Could you check a few things on this model? Use its own coordinates, in mm. A direction names the side the tool comes from. Round coordinates to 2 decimals unless told otherwise and drop trailing zeros. Use CSV: the item, a comma, the result in double quotes. Start each with the question number.
Autodesk Inventor part; units mm, degrees
ref_plane "Work Plane1" through (-41.275, 69.85, 0) normal (0, -1, 0) x (0, 0, -1)
ref_plane "YZ Plane" through (0, 0, 0) normal (1, 0, 0) x (0, 1, 0)
ref_plane "XZ Plane" through (0, 0, 0) normal (0, 1, 0) x (-1, 0, 0)
sketch "Sketch1" plane through (0, 0, 0) normal (0, 0, 1) x (1, 0, 0)
  line L0 (-47.625, -69.85) -> (47.625, -69.85)
  line L1 (47.625, -69.85) -> (47.625, 69.85)
  line L2 (47.625, 69.85) -> (-47.625, 69.85)
  line L3 (-47.625, 69.85) -> (-47.625, -69.85)
  line L4 (-47.625, -69.85) -> (47.625, 69.85) construction
  line L5 (47.625, -69.85) -> (-47.625, 69.85) construction
  point P0 (0, 0)
  dimension "d2" = 95.25
  dimension "d3" = 139.7
extrude "Extrusion1" add sketch "Sketch1" along normal blind 12.7
sketch "Sketch5" plane through (0, 0, 0) normal (0, 0, -1) x (-1, 0, 0)
  circle A0 centre (68.072, -112.9665) radius 2.5527
  circle A1 centre (17.272, -112.9665) radius 2.5527
  circle A2 centre (-33.528, -112.9665) radius 2.5527
  circle A3 centre (-84.328, -112.9665) radius 2.5527
  circle A4 centre (-135.128, -112.9665) radius 2.5527
  circle A5 centre (-185.928, -112.9665) radius 2.5527
  circle A6 centre (-211.328, -112.9665) radius 2.5527
  circle A7 centre (-160.528, -112.9665) radius 2.5527
  circle A8 centre (-109.728, -112.9665) radius 2.5527
  circle A9 centre (-58.928, -112.9665) radius 2.5527
  circle A10 centre (-8.128, -112.9665) radius 2.5527
  circle A11 centre (42.672, -112.9665) radius 2.5527
  circle A12 centre (93.472, -112.9665) radius 2.5527
  circle A13 centre (-62.484, -38.6715) radius 3.429
  circle A14 centre (-62.484, 33.7185) radius 3.429
  arc A15 (-54.102, -15.1765) -> (-44.45, -15.1765) centre (-49.276, -15.1765) ccw
  line L0 (-44.45, -15.1765) -> (-44.45, 10.2235)
  arc A16 (-44.45, 10.2235) -> (-54.102, 10.2235) centre (-49.276, 10.2235) ccw
  line L1 (-54.102, 10.2235) -> (-54.102, -15.1765)
  arc A17 (-228.854, -15.1765) -> (-219.202, -15.1765) centre (-224.028, -15.1765) ccw
  line L2 (-219.202, -15.1765) -> (-219.202, 10.2235)
  arc A18 (-219.202, 10.2235) -> (-228.854, 10.2235) centre (-224.028, 10.2235) ccw
  line L3 (-228.854, 10.2235) -> (-228.854, -15.1765)
  circle A19 centre (-218.3546, -258.6355) radius 2.413
  circle A20 centre (-78.4098, -256.2225) radius 2.413
  circle A21 centre (-78.4098, -297.1165) radius 2.413
  circle A22 centre (-218.3546, -294.7035) radius 2.413
  circle A23 centre (112.522, -87.5665) radius 2.0701
  circle A24 centre (112.522, -138.3665) radius 2.0701
  circle A25 centre (-243.078, 64.8335) radius 2.0701
  circle A26 centre (-243.078, 14.0335) radius 2.0701
  circle A27 centre (-243.078, -36.7665) radius 2.0701
  circle A28 centre (-243.078, -87.5665) radius 2.0701
  circle A29 centre (-243.078, -138.3665) radius 2.0701
  circle A30 centre (-243.078, -189.1665) radius 2.0701
  circle A31 centre (-243.078, -239.9665) radius 2.0701
  circle A32 centre (-243.078, -290.7665) radius 2.0701
  circle A33 centre (-243.078, -265.3665) radius 2.0701
  circle A34 centre (-243.078, -214.5665) radius 2.0701
  circle A35 centre (-243.078, -163.7665) radius 2.0701
  circle A36 centre (-243.078, -112.9665) radius 2.0701
  circle A37 centre (-243.078, -62.1665) radius 2.0701
  circle A38 centre (-243.078, -11.3665) radius 2.0701
  circle A39 centre (-243.078, 39.4335) radius 2.0701
  circle A40 centre (112.522, -163.7665) radius 2.0701
  circle A41 centre (112.522, -112.9665) radius 2.0701
  circle A42 centre (112.522, -62.1665) radius 2.0701
  arc A43 (-45.1979, 77.5335) -> (-51.5479, 83.8835) centre (-51.5479, 77.5335) ccw
  line L4 (-45.1979, 77.5335) -> (-45.1979, 54.7638)
  arc A44 (-45.1979, 54.7638) -> (-43.3381, 50.2736) centre (-38.8479, 54.7638) ccw
  line L5 (-43.3381, 50.2736) -> (29.1422, -22.2066)
  arc A45 (31.0021, -26.6968) -> (29.1422, -22.2066) centre (24.6521, -26.6968) ccw
  line L6 (31.0021, -26.6968) -> (31.0021, -43.1165)
  arc A46 (31.0021, -43.1165) -> (37.3521, -49.4665) centre (37.3521, -43.1165) ccw
  line L7 (37.3521, -49.4665) -> (118.872, -49.4665)
  line L8 (118.872, -176.4665) -> (118.872, -49.4665)
  line L9 (118.872, -176.4665) -> (37.3521, -176.4665)
  arc A47 (37.3521, -176.4665) -> (31.0021, -182.8165) centre (37.3521, -182.8165) ccw
  line L10 (31.0021, -182.8165) -> (31.0021, -199.2362)
  arc A48 (29.1422, -203.7264) -> (31.0021, -199.2362) centre (24.6521, -199.2362) ccw
  line L11 (29.1422, -203.7264) -> (-43.3381, -276.2066)
  arc A49 (-43.3381, -276.2066) -> (-45.1979, -280.6968) centre (-38.8479, -280.6968) ccw
  line L12 (-45.1979, -280.6968) -> (-45.1979, -303.4665)
  arc A50 (-51.5479, -309.8165) -> (-45.1979, -303.4665) centre (-51.5479, -303.4665) ccw
  line L13 (-249.428, -309.8165) -> (-51.5479, -309.8165)
  line L14 (-249.428, 83.8835) -> (-249.428, -309.8165)
  line L15 (-51.5479, 83.8835) -> (-249.428, 83.8835)
  line L16 (-47.625, -69.85) -> (-47.625, 69.85)
  line L17 (47.625, 69.85) -> (47.625, -69.85)
  line L18 (47.625, -69.85) -> (-47.625, -69.85)
  line L19 (28.575, 28.5877) -> (-28.575, 28.5877)
  circle A51 centre (19.05, -44.45) radius 3.3782
  circle A52 centre (-22.225, 19.0627) radius 3.3782
  point P0 (0, 0)
  point P1 (22.225, -38.1)
  point P2 (-25.4, 19.0627)
  point P3 (20.684, -69.85)
  point P4 (-44.45, 19.0627)
  point P5 (19.05, -69.85)
  point P6 (-3.175, -15.875)
  dimension "d47" = 25.4
  dimension "d53" = 22.225
  dimension "d64" = 19.0627
  dimension "d65" = 38.1
  dimension "d108" = 25.4
  dimension "d109" = 53.975
hole "Hole1" at (-22.225, -38.1, 0) at (25.4, 19.0627, 0) at (3.175, -15.875, 0) direction (0, 0, 1) diameter 5.1054 end through all
ref_plane "Work Plane1" through (-41.275, 69.85, 0) normal (0, -1, 0) x (0, 0, -1)
sketch "Sketch7" plane through (0, 0, 12.7) normal (0, 0, 1) x (1, 0, 0)
  line L0 (-9.525, -69.85) -> (47.625, 11.7687)
  line L1 (-47.625, -69.85) -> (47.625, -69.85)
  line L2 (-47.625, 69.85) -> (-47.625, -69.85)
  line L3 (47.625, -69.85) -> (47.625, 69.85)
  line L4 (47.625, 69.85) -> (-47.625, 69.85)
  line L5 (27.625, 69.85) -> (-30.7357, 69.85)
  line L6 (-30.7357, 69.85) -> (-30.7357, 28.5877)
  line L7 (-30.7357, 28.5877) -> (27.625, 28.5877)
  line L8 (-16.7842, 38.1127) -> (14.9658, 38.1127)
  line L9 (-16.7842, 50.8127) -> (14.9658, 50.8127)
  line L10 (14.9658, 50.8127) -> (14.9658, 38.1127)
  line L11 (-16.7842, 50.8127) -> (-16.7842, 38.1127)
  line L12 (20.4436, 50.8127) -> (24.45, 50.8127)
  line L13 (24.0601, 50.8127) -> (24.45, 50.8127)
  line L14 (24.0601, 50.8127) -> (-14.952, 50.8127)
  line L15 (20.4436, 50.8127) -> (17.9874, 50.8127)
  line L16 (-2.2262, 50.8127) -> (17.9874, 50.8127)
  line L17 (-2.2262, 52.3875) -> (17.9874, 52.3875)
  line L18 (17.9874, 52.3875) -> (20.4436, 52.3875)
  line L19 (20.4436, 52.3875) -> (24.45, 52.3875)
  line L20 (24.45, 50.8127) -> (24.45, 52.3875)
  line L21 (-21.2107, 52.3875) -> (-9.8426, 52.3875)
  line L22 (-9.8426, 52.3875) -> (-7.673, 52.3875)
  line L23 (-7.673, 52.3875) -> (-5.0722, 52.3875)
  line L24 (-5.0722, 52.3875) -> (-2.2262, 52.3875)
  line L25 (27.625, 28.5877) -> (27.625, 69.85)
  dimension "d72" = 9.525
  dimension "d73" = 3.175
  dimension "d74" = 9.525
  dimension "d80" = 38.1
  dimension "d84" = 55
extrude "Extrusion7" cut sketch "Sketch7" against normal blind 11.1125 contours L25 L7 L6 L4 | L11 L9 L10 L8
extrude "Extrusion9" cut sketch "Sketch7" against normal through all contours L0 L3 L1
chamfer "Chamfer3" distance 12.7 angle 45 4 edges at (47.625, 40.8093, 0) (19.05, -29.0407, 0) (-47.625, 0, 0) (-28.575, -69.85, 0)
sketch "Sketch8" plane through (0, 0, 0) normal (0, 0, -1) x (-1, 0, 0)
  line L0 (16.1925, 52.07) -> (13.0175, 52.07) construction
  line L1 (16.1925, 55.4482) -> (13.0175, 55.4482)
  line L2 (13.0175, 48.6918) -> (16.1925, 48.6918)
  arc A0 (16.1925, 48.6918) -> (16.1925, 55.4482) centre (16.1925, 52.07) ccw
  arc A1 (13.0175, 55.4482) -> (13.0175, 48.6918) centre (13.0175, 52.07) ccw
  line L3 (34.925, 69.85) -> (34.925, -57.15)
  line L4 (-34.925, 69.85) -> (34.925, 69.85)
  point P0 (0, 0)
  point P1 (14.605, 52.07)
  dimension "d88" = 3.3782
  dimension "d89" = 3.175
  dimension "d90" = 20.32
  dimension "d91" = 17.78
extrude "Extrusion10" cut sketch "Sketch8" against normal blind 11.1125
sketch "Sketch10" plane through (0, 0, 12.7) normal (0, 0, 1) x (1, 0, 0)
  line L0 (-9.525, -69.85) -> (47.625, 11.7687)
  line L1 (47.625, 11.7687) -> (47.625, 69.85)
  line L2 (47.625, 69.85) -> (27.625, 69.85)
  line L3 (27.625, 69.85) -> (27.625, 28.5877)
  line L4 (27.625, 28.5877) -> (-30.7357, 28.5877)
  line L5 (-30.7357, 28.5877) -> (-30.7357, 69.85)
  line L6 (-30.7357, 69.85) -> (-47.625, 69.85)
  line L7 (-47.625, 69.85) -> (-47.625, -69.85)
  line L8 (-47.625, -69.85) -> (-9.525, -69.85)
  circle A0 centre (25.4, 19.0627) radius 2.5527
  circle A1 centre (-22.225, -38.1) radius 2.5527
  circle A2 centre (3.175, -15.875) radius 2.5527
  arc A3 (-13.0175, 48.6918) -> (-13.0175, 55.4482) centre (-13.0175, 52.07) ccw
  line L9 (-13.0175, 48.6918) -> (-16.1925, 48.6918)
  arc A4 (-16.1925, 55.4482) -> (-16.1925, 48.6918) centre (-16.1925, 52.07) ccw
  line L10 (-16.1925, 55.4482) -> (-13.0175, 55.4482)
  line L11 (-30.7357, 69.85) -> (27.625, 69.85)
  line L12 (-30.7357, 28.5877) -> (-30.7357, 69.85)
  line L13 (27.625, 28.5877) -> (-30.7357, 28.5877)
  line L14 (27.625, 69.85) -> (27.625, 28.5877)
  point P0 (0, 0)
properties part number "C34_TK_UnderCarriageGuardPlate" material "Polycarbonate, Clear"
1. We'd pull the mould along X, two halves only. Please class faces 4 (the face through (-41.186, -0.978, 6.261)), 5 (the face through (4.153, -13.517, 6.439)), 6 (the face through (14.32, -24.88, 6.44)), 7 (the face through (1, 69.85, 1)): pulls with the +X half, pulls with the -X half, needs draft (parallel to the pull), parting line crosses it, or undercut.
2. Suppose I cut it at B-B (z = 8.5). State how many separate pieces and enclosed holes the cut face has, then the cut area to 3 significant figures.
3. Will these pins go through, and if not, where does the flat tip stop? pin 1 (5.5 mm diameter, centred on y = 46, z = 6.5, fed in from -X); pin 2 (3 mm diameter, centred on y = -12.5, z = 5.5, fed in from +X); pin 3 (2 mm diameter, centred on x = 20.5, z = 5.5, fed in from +Y).
4. For faces 1 (the face through (41.364, 40.403, 6.439)), 2 (the face through (-2, 28.588, 7)), 3 (the face through (-19.57, 52, 0.78)), which set-ups out of +Z, -Z, +X, -X, +Y, -Y let a thin tool reach every point of the face, with its end or its side?
5. If I drill on L1, parallel to Y at x = 25.4, z = 6.5; L2, parallel to Z at x = 10.5, y = 58.5; L3, parallel to Z at x = -36.5, y = 60, over which ranges is the centre line in solid material (lowest first)?
Geometry check:
1,face 4,"pulls with the -X half"
1,face 5,"undercut"
1,face 6,"pulls with the +X half"
1,face 7,"needs draft"
2,separate pieces,"1"
2,enclosed holes,"3"
2,area,"7,130 mm²"
3,pin 1,"stops at x = -44.18"
3,pin 2,"stops at x = 23.95"
3,pin 3,"stops at y = 28.59"
4,face 1,"-Z, +X, +Y, -Y"
4,face 2,"+Z, +Y"
4,face 3,"+Z, -Z"
5,L1,"y = -9.16 to 16.51, 21.62 to 28.59"
5,L2,"z = 0 to 1.59"
5,L3,"z = 1.57 to 12.7"
